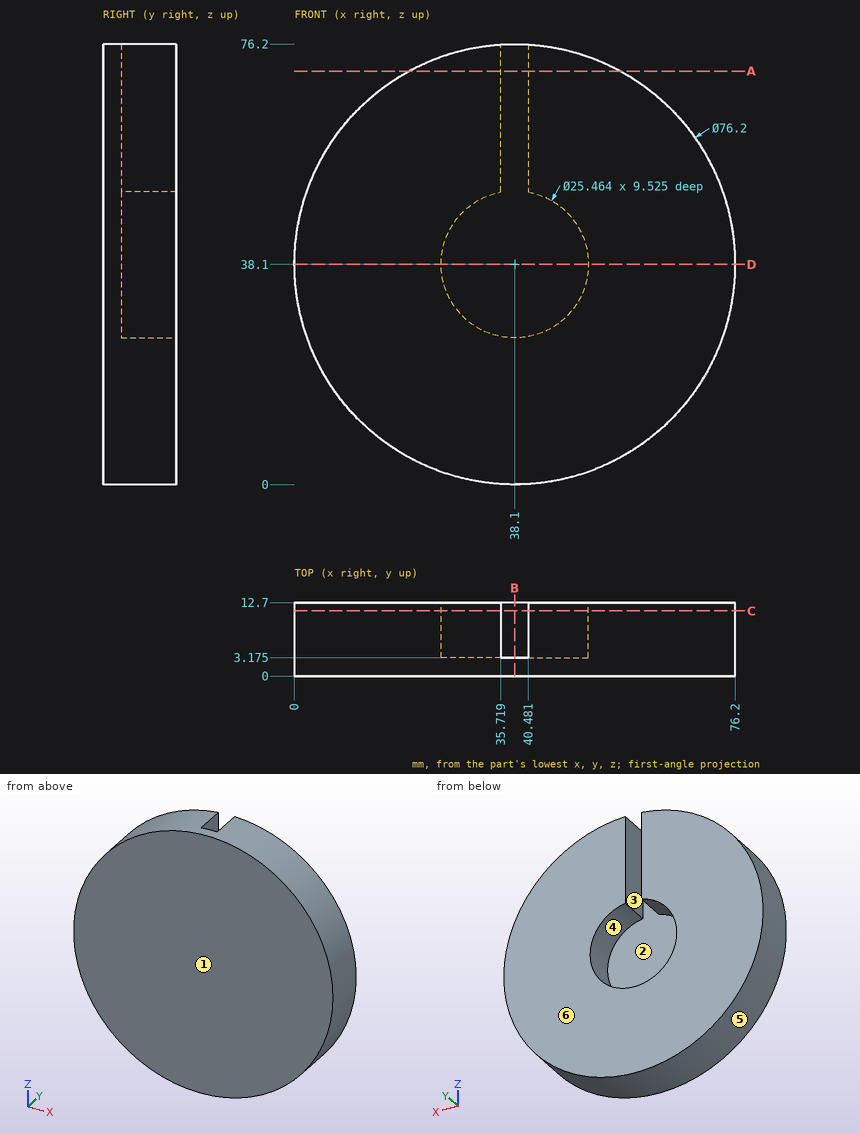
Here's the drawing with two shaded views (mm, measured from the low corner). I have some questions. A direction names the side the tool comes from. Round coordinates to 2 decimals unless told otherwise and drop trailing zeros. Order: outer loops, then holes, each group sorted by start corner. A loop starts at its lowest first (then second) coordinate and runs counter-clockwise, first axis right, second up. Notation, with made-up numbers: M 36.5,41.5 L 49.5,41.5 A16 ccw 49.5,66.5 Z; hole C 15,-8.75 d8. An arc over 180 degrees is marked long. Answer in a Markdown table with one row per item.
Item 1: Imagine slicing it at D-D, the plane z = 38.1. Write out the boundary of the cut face in (x, y) (1 decimal), and give its area (3 significant figures).
A:
| item | result |
|---|---|
| outline | M 0,0 L 76.2,0 L 76.2,12.7 L 50.8,12.7 L 50.8,3.2 L 25.4,3.2 L 25.4,12.7 L 0,12.7 Z |
| area | 725 mm2 |
Item 2: For the marked faces 1, 2 and 3, which set-ups out of +Z, -Z, +X, -X, +Y, -Y let a thin tool reach every point of the face, with its end or its side?
A:
| item | result |
|---|---|
| face 1 | +Z, -Z, +X, -X, -Y |
| face 2 | +Y |
| face 3 | +Z, +Y |
Item 3: If I drill on L1, parallel to X at y = 5.25, z = 38.1; L2, parallel to X at y = 4.5, z = 64.5; L3, parallel to Z at x = 46, y = 11 (1 decimal), over which ranges is the centre line in solid material (lowest first)? Write a range as from..to.
A:
| item | result |
|---|---|
| L1 | x = 0..25.37, 50.83..76.2 |
| L2 | x = 10.63..35.72, 40.48..65.57 |
| L3 | z = 0.8..28.1, 48.1..75.4 |
Item 4: Imagine slicing it at B-B, the plane x = 38.1. Write out the boundary of the cut face in (y, z) (1 decimal).
A:
| item | result |
|---|---|
| outline | M 0,0 L 12.7,0 L 12.7,25.4 L 3.2,25.4 L 3.2,76.2 L 0,76.2 Z |
Item 5: Thinking about a two-plate mould opening in X: for the marked faces 4, 5 and 6, which applies, +X half, -X half, draft (parallel to the pull), parting line (faces both ways), or undercut?
A:
| item | result |
|---|---|
| face 4 | undercut |
| face 5 | parting line |
| face 6 | draft |
Item 6: Imagine slicing it at A-A, the plane z = 71.5. Write out the boundary of the cut face in (x, y) (1 decimal).
A:
| item | result |
|---|---|
| outline | M 19.8,0 L 56.4,0 L 56.4,12.7 L 40.5,12.7 L 40.5,3.2 L 35.7,3.2 L 35.7,12.7 L 19.8,12.7 Z |
Item 7: I'm going to push flat-ended pins straight in: pin 1 (6 mm diameter, centred on x = 64, y = 5, fed in from +Z); pin 2 (2 mm diameter, centred on y = 9.5, z = 33.5, fed in from +X); pin 3 (7.5 mm diameter, centred on x = 38.5, z = 46, fed in from +Y) (1 decimal). Where does each tip first touch, or does it pass through?
A:
| item | result |
|---|---|
| pin 1 | stops at z = 68.55 |
| pin 2 | stops at x = 76.03 |
| pin 3 | stops at y = 3.2 |
Item 8: Imagine slicing it at C-C, the plane y = 11.25. Write out the boundary of the cut face in (x, z) (1 decimal).
A:
| item | result |
|---|---|
| outline | M 35.7,50.6 L 35.7,76.1 A38.1 ccw long 40.5,76.1 L 40.5,50.6 A12.7 cw long Z |
